Geometry: final body of the model. Coordinates: model frame, mm. A direction names the side the tool comes from. Coordinates: 2 decimals unless noted, no trailing zeros. Order: outer loops, then holes, each group sorted by start corner. A loop starts at its lowest first (then second) coordinate and runs counter-clockwise, first axis right, second up. Notation, with made-up numbers: (-35, -23.75) -> (4, -23.75) arc R14 ccw to (4, -14.75) -> close; hole circle Ø10 at (-13.75, 13). An arc over 180 degrees is marked (long way). Use one line per item in the form item = value.
Autodesk Inventor part; units mm, degrees
ref_plane "YZ Plane" through (0, 0, 0) normal (1, 0, 0) x (0, 1, 0)
ref_plane "XZ Plane" through (0, 0, 0) normal (0, 1, 0) x (-1, 0, 0)
ref_plane "XY Plane" through (0, 0, 0) normal (0, 0, 1) x (1, 0, 0)
sketch "Sketch1" plane through (0, 0, 0) normal (0, 1, 0) x (-1, 0, 0)
  line L0 (101.6, 38.1) -> (-101.6, 38.1) construction
  line L1 (-101.6, 38.1) -> (-101.6, -38.1) construction
  line L2 (-101.6, -38.1) -> (101.6, -38.1) construction
  line L3 (101.6, -38.1) -> (101.6, 38.1) construction
  line L4 (101.6, 38.1) -> (-101.6, -38.1) construction
  line L5 (-101.6, 38.1) -> (101.6, -38.1) construction
  line L6 (-28.575, 66.675) -> (28.575, 66.675) construction
  line L7 (28.575, 66.675) -> (28.575, 9.525)
  line L8 (28.575, 9.525) -> (-28.575, 9.525) construction
  line L9 (-28.575, 9.525) -> (-28.575, 66.675)
  line L10 (-28.575, 66.675) -> (28.575, 9.525) construction
  line L11 (28.575, 66.675) -> (-28.575, 9.525) construction
  circle A0 centre (-38.1, 50.8) radius 3.175
  line L12 (0, 38.1) -> (0, -38.1) construction
  circle A1 centre (-38.1, 50.8) radius 9.525
  line L13 (-38.1, 60.325) -> (-28.575, 60.325)
  circle A2 centre (38.1, 50.8) radius 3.175
  circle A3 centre (38.1, 50.8) radius 9.525
  line L14 (38.1, 60.325) -> (28.575, 60.325)
  circle A4 centre (-76.2, -38.1) radius 1.7526
  circle A5 centre (-95.25, 3.175) radius 1.7526
  circle A6 centre (76.2, -38.1) radius 1.7526
  circle A7 centre (95.25, 3.175) radius 1.7526
  line L15 (-101.6, -38.1) -> (-101.6, 6.35)
  line L16 (-101.6, 6.35) -> (-44.4797, 57.8728)
  line L17 (101.6, -38.1) -> (101.6, 6.35)
  line L18 (101.6, 6.35) -> (44.4797, 57.8728)
  line L19 (-42.6417, 42.4275) -> (-86.025, 3.2956) construction
  line L20 (-86.025, 3.2956) -> (-86.025, -38.1)
  line L21 (86.025, -38.1) -> (86.025, 3.2956)
  line L22 (86.025, 3.2956) -> (42.6417, 42.4275) construction
  line L23 (0, -38.1) -> (-95.25, -38.1) construction
  line L24 (0, -38.1) -> (95.25, -38.1) construction
  circle A8 centre (-60.325, 35.0287) radius 1.7526
  circle A9 centre (-33.3375, 31.75) radius 1.7526
  line L25 (-38.1, 0) -> (-38.1, 41.275)
  line L26 (-38.1, 0) -> (0, 0) construction
  circle A10 centre (60.325, 35.0287) radius 1.7526
  circle A11 centre (33.3375, 31.75) radius 1.7526
  line L27 (38.1, 0) -> (38.1, 41.275)
  line L28 (38.1, 0) -> (0, 0) construction
  line L29 (-86.025, 0) -> (-60.1, 0)
  line L30 (-60.1, 0) -> (-60.1, -31.75)
  line L31 (-60.1, -31.75) -> (-87.975, -31.75)
  line L32 (-101.6, -38.1) -> (101.6, -38.1) construction
  line L33 (101.6, -38.1) -> (101.6, 19.05)
  line L34 (101.6, 19.05) -> (-101.6, 19.05) construction
  line L35 (-101.6, 19.05) -> (-101.6, -38.1)
  line L36 (-101.6, 19.05) -> (-87.5203, 19.05) construction
  line L37 (87.5203, 19.05) -> (101.6, 19.05) construction
  circle A12 centre (-38.1, 0) radius 3.175 construction
  circle A13 centre (-38.1, 0) radius 6.35 construction
  circle A14 centre (38.1, 0) radius 3.175 construction
  circle A15 centre (38.1, 0) radius 6.35 construction
  circle A16 centre (28.575, 9.525) radius 1.7526
  circle A17 centre (28.575, 9.525) radius 4.7625
  arc A18 (17.0773, 9.525) -> (28.575, 21.0227) centre (17.0773, 21.0227) ccw
  circle A19 centre (-28.575, 9.525) radius 1.7526
  circle A20 centre (-28.575, 9.525) radius 4.7625
  arc A21 (-28.575, 21.0227) -> (-17.0773, 9.525) centre (-17.0773, 21.0227) ccw
  arc A22 (31.4325, 5.715) -> (38.1, 19.05) centre (21.4312, 19.05) ccw
  arc A23 (-38.1, 19.05) -> (-31.4325, 5.715) centre (-21.4312, 19.05) ccw
  line L38 (-56.925, -38.1) -> (-56.925, 29.544)
  line L39 (86.025, 0) -> (60.1, 0)
  line L40 (60.1, 0) -> (60.1, -31.75)
  line L41 (60.1, -31.75) -> (87.975, -31.75)
  line L42 (56.925, -38.1) -> (56.925, 29.544)
  line L43 (-28.575, 4.7625) -> (28.575, 4.7625)
  line L44 (101.6, -31.75) -> (-101.6, -31.75)
  line L45 (-101.6, -31.75) -> (-101.6, -44.45) construction
  line L46 (-101.6, -44.45) -> (101.6, -44.45)
  line L47 (101.6, -44.45) -> (101.6, -31.75) construction
  circle A24 centre (0, -38.1) radius 1.7526
  circle A25 centre (38.1, -38.1) radius 1.7526
  circle A26 centre (-38.1, -38.1) radius 1.7526
  line L48 (101.6, -38.1) -> (76.2, -44.45)
  line L49 (-101.6, -38.1) -> (-76.2, -44.45)
  line L50 (76.2, -38.1) -> (76.2, -44.45) construction
  line L51 (-76.2, -38.1) -> (-76.2, -44.45) construction
  line L52 (59.1924, 41.2769) -> (32.488, 36.4361)
  circle A27 centre (60.325, 35.0287) radius 6.35
  circle A28 centre (33.3375, 31.75) radius 4.7625
  line L53 (-59.1924, 41.2769) -> (-32.488, 36.4361)
  circle A29 centre (-60.325, 35.0287) radius 6.35
  circle A30 centre (-33.3375, 31.75) radius 4.7625
  line L54 (-86.025, 0) -> (-60.1, 0)
  line L55 (-60.1, 0) -> (-60.1, -3.175)
  line L56 (-60.1, -3.175) -> (-86.025, -3.175)
  line L57 (-86.025, -3.175) -> (-86.025, 0)
  line L58 (-60.1, -15.875) -> (-86.025, -15.875) construction
  line L59 (-60.1, -28.575) -> (-86.025, -28.575)
  line L60 (-82.85, -38.1) -> (-82.85, 0.1248)
  line L61 (60.1, -3.175) -> (86.025, -3.175)
  line L62 (60.1, -15.875) -> (86.025, -15.875) construction
  line L63 (60.1, -28.575) -> (86.025, -28.575)
  line L64 (82.85, -38.1) -> (82.85, 0.1248)
  line L65 (-33.3375, -31.75) -> (33.3375, -31.75)
  line L66 (33.3375, -31.75) -> (33.3375, 3.175) construction
  line L67 (33.3375, 3.175) -> (-33.3375, 3.175)
  line L68 (-33.3375, 3.175) -> (-33.3375, -31.75) construction
  circle A31 centre (41.275, 25.4) radius 3.175
  circle A32 centre (-41.275, 25.4) radius 3.175
  line L69 (-17.0773, 9.525) -> (17.0773, 9.525)
  line L70 (0, -31.75) -> (-41.275, -31.75)
  line L71 (-41.275, -31.75) -> (-33.3375, 3.175)
  line L72 (41.275, -31.75) -> (33.3375, 3.175)
  point P0 (28.575, 38.1)
  point P1 (-28.575, 38.1)
  point P2 (28.575, 60.325)
  point P3 (44.4797, 57.8728)
  point P4 (101.6, -15.875)
  point P5 (38.1, 41.275)
  point P6 (-86.025, -31.75)
  point P7 (-101.6, 6.35)
  point P8 (101.6, 6.35)
  point P9 (31.75, 0)
  point P10 (38.1, 6.35)
  point P11 (-38.1, 6.35)
  point P12 (-31.75, 0)
  point P13 (86.025, -31.75)
  point P14 (56.925, 29.544)
  point P15 (-17.0773, 9.525)
  point P16 (-28.575, 21.0227)
  point P17 (-38.1, 19.05)
  point P18 (-31.4325, 5.715)
  point P19 (-21.8502, 0)
  point P20 (21.8502, 0)
  point P21 (-25.2074, 12.8926)
  point P22 (-28.575, 14.2875)
  point P23 (-23.8125, 9.525)
  point P24 (-28.575, 50.8)
  point P25 (25.2074, 12.8926)
  point P26 (28.575, 14.2875)
  point P27 (23.8125, 9.525)
  point P28 (28.575, 50.8)
  point P29 (26.8224, 9.525)
  point P30 (28.575, 11.2776)
  point P31 (56.925, -31.75)
  point P32 (-56.925, -31.75)
  point P33 (-28.575, 31.75)
  point P34 (-64.5781, 39.7439)
  point P35 (64.5781, 39.7439)
  point P36 (28.575, 31.75)
  point P37 (-82.85, -3.175)
  point P38 (-60.1, -28.575)
  point P39 (-82.85, -28.575)
  point P40 (60.1, -3.175)
  point P41 (82.85, -3.175)
  point P42 (82.85, -28.575)
  point P43 (60.1, -28.575)
  point P44 (33.3375, -31.75)
  point P45 (86.025, -31.75)
  point P46 (-86.025, -31.75)
  point P47 (-60.1, -31.75)
  point P48 (-101.6, -31.75)
  point P49 (-26.8224, 9.525)
  point P50 (-28.575, 11.2776)
  point P51 (-39.8526, -38.1)
  point P52 (-36.3474, -38.1)
  point P53 (-1.7526, -38.1)
  point P54 (1.7526, -38.1)
  point P55 (36.3474, -38.1)
  point P56 (39.8526, -38.1)
  point P57 (-60.1, -31.75)
  point P58 (-87.975, -31.75)
  point P59 (41.275, -31.75)
  dimension "d0" = 203.2
  dimension "d1" = 76.2
  dimension "d4" = 57.15
  dimension "d6" = 6.35
  dimension "d7" = 38.1
  dimension "d8" = 19.05
  dimension "d10" = 3.5052
  dimension "d11" = 3.5052
  dimension "d12" = 0
  dimension "d14" = 25.4
  dimension "d15" = 6.35
  dimension "d20" = 50.8
  dimension "d21" = 41.275
  dimension "d22" = 44.45
  dimension "d24" = 12.7
  dimension "d25" = 15.575
  dimension "d26" = 12.7
  dimension "d27" = 15.575
  dimension "d31" = 3.5052
  dimension "d32" = 3.5052
  dimension "d33" = 6.35
  dimension "d34" = 31.75
  dimension "d35" = 4.7625
  dimension "d36" = 22.225
  dimension "d37" = 9.525
  dimension "d39" = 31.75
  dimension "d40" = 6.35
  dimension "d42" = 57.15
  dimension "d43" = 6.35
  dimension "d44" = 9.525
  dimension "d45" = 9.525
  dimension "d46" = 12.7
  dimension "d104" = 3.5052
  dimension "d105" = 9.525
  dimension "d106" = 3.175
  dimension "d123" = 88.9
  dimension "d124" = 12.7
  dimension "d125" = 3.5052
  dimension "d126" = 3.5052
  dimension "d127" = 38.1
  dimension "d128" = 28.575
  dimension "d129" = 3.175
  dimension "d130" = 3.175
  dimension "d131" = 33.3375
  dimension "d132" = 33.3375
  dimension "d133" = 34.925
  dimension "d135" = 6.35
  dimension "d138" = 6.35
  dimension "d139" = 3.175
  dimension "d140" = 41.275
  dimension "d144" = 41.5
extrude "Extrusion1" add sketch "Sketch1" along normal blind 3.175 contours A28 L27 A22 A17 L7 | A28 | L7 A17 A18 | L52 L27 A28 | L27 L52 A27 L18 L17 L44 L41 L21 L39 L40 L72 L67 L71 L30 L29 L20 L31 L15 L16 A29 L53 L25 A23 A20 L43 A17 A22 | A27 | A17 | A17 L43 A20 A21 L69 A18 | L17 L48 L46 L49 L15 L44 L31 L41 | A20 | A23 L25 A30 L9 A20 | A20 L9 A21 | L41 L64 L63 L21 | L63 L64 L61 L21 | L41 L40 L63 L64 | A30 | L61 L64 L39 L21 | L25 L53 A30 | L61 L40 L39 L64 | A29 | L20 L59 L60 L31 | L20 L56 L60 L59 | L60 L59 L30 L31 | L20 L29 L60 L56 | L60 L29 L30 L56
fillet "Fillet1" radius 6.35 6 edges at (101.6, 1.5875, -38.1) (101.6, 1.5875, 6.35) (-101.6, 1.5875, 6.35) (76.2, 1.5875, -44.45) (-76.2, 1.5875, -44.45) (-101.6, 1.5875, -38.1)
fillet "Fillet5" radius 3.175 4 edges at (33.3375, 1.5875, 3.175) (-33.3375, 1.5875, 3.175) (-41.275, 1.5875, -31.75) (41.275, 1.5875, -31.75)
fillet "Fillet6" radius 4.7625 8 edges at (-82.85, 1.5875, -28.575) (-60.1, 1.5875, -28.575) (-60.1, 1.5875, -3.175) (-82.85, 1.5875, -3.175) (60.1, 1.5875, -28.575) (82.85, 1.5875, -28.575) (60.1, 1.5875, -3.175) (82.85, 1.5875, -3.175)
equation "\"d35\" = 0.5 * d37"
properties part number "Chassis" material "UHMW, White"
1) Pull-direction query (X, two-part tool) for faces 4 (the cylindrical face through (-61.532, 1.61, -4.533)), 5 (the flat face through (1, 0, 9)), 6 (the flat face through (82.29, 1.57, 23.77)), 7 (the cylindrical face through (44.447, 1.565, 25.26)); classes: released by +X, released by -X, zero draft, split by the parting line, or undercut.
Results found:
face_4 = undercut
face_5 = zero draft
face_6 = released by +X
face_7 = undercut
2) Section A-A, the plane z = -13. Output: boundary loops of the cut face in (x, y) (3 decimals), and give its area (3 significant figures).
Results found:
outline = (-101.6, 0) -> (-82.85, 0) -> (-82.85, 3.175) -> (-101.6, 3.175) -> close; (-60.1, 0) -> (-37.014, 0) -> (-37.014, 3.175) -> (-60.1, 3.175) -> close; (37.014, 0) -> (60.1, 0) -> (60.1, 3.175) -> (37.014, 3.175) -> close; (82.85, 0) -> (101.6, 0) -> (101.6, 3.175) -> (82.85, 3.175) -> close
area = 266 mm2
3) Section C-C, the plane y = 1.8. Give the number of separate pieces and of enclosed holes in the cut face, and give its area (3 significant figures).
Results found:
separate_pieces = 1
enclosed_holes = 18
area = 10,100 mm2
4) Section B-B, the plane x = 19. Output: boundary loops of the cut face in (y, z) (3 decimals), and give its area (3 significant figures).
Results found:
outline = (0, -44.45) -> (3.175, -44.45) -> (3.175, -31.75) -> (0, -31.75) -> close; (0, 3.175) -> (3.175, 3.175) -> (3.175, 9.687) -> (0, 9.687) -> close
area = 61.0 mm2
5) Contact query for a flat-ended pin moving along its axis: P1, Ø1, axis at x = 11, y = 1.5, coming from the +Z side (3 decimals). Output: stop coordinate, or through.
Results found:
P1 = 9.525
6) Access query for faces 1 (the cylindrical face through (-61.458, 1.61, -27.143)), 2 (the cylindrical face through (100.291, 1.61, -37.003)), 3 (the flat face through (46.03, 1.57, 38.89)). Directions: +Z, -Z, +X, -X, +Y, -Y. A direction counts if a zero-diameter tool reaches every point of the face in a straight line with its end or side. Return the directions, or none.
Results found:
face_1 = +Y, -Y
face_2 = -Z, +X, +Y, -Y
face_3 = +Z, +Y, -Y
7) Section D-D, the plane x = 49.5. Output: boundary loops of the cut face in (y, z) (3 decimals).
Results found:
outline = (0, -44.45) -> (3.175, -44.45) -> (3.175, 39.52) -> (0, 39.52) -> close
8) Material intervals for probe 1 along Z at (x, y) = (0, 0.75) (3 decimals); probe 2 along Z at (x, y) = (7, 1.4) (3 decimals); probe 3 along Z at (x, y) = (-0.5, 1.85) (3 decimals), sorted ascending. Write a range as from..to.
Results found:
probe_1 = -44.45..-39.853, -36.347..-31.75, 3.175..9.525
probe_2 = -44.45..-31.75, 3.175..9.525
probe_3 = -44.45..-39.78, -36.42..-31.75, 3.175..9.525
